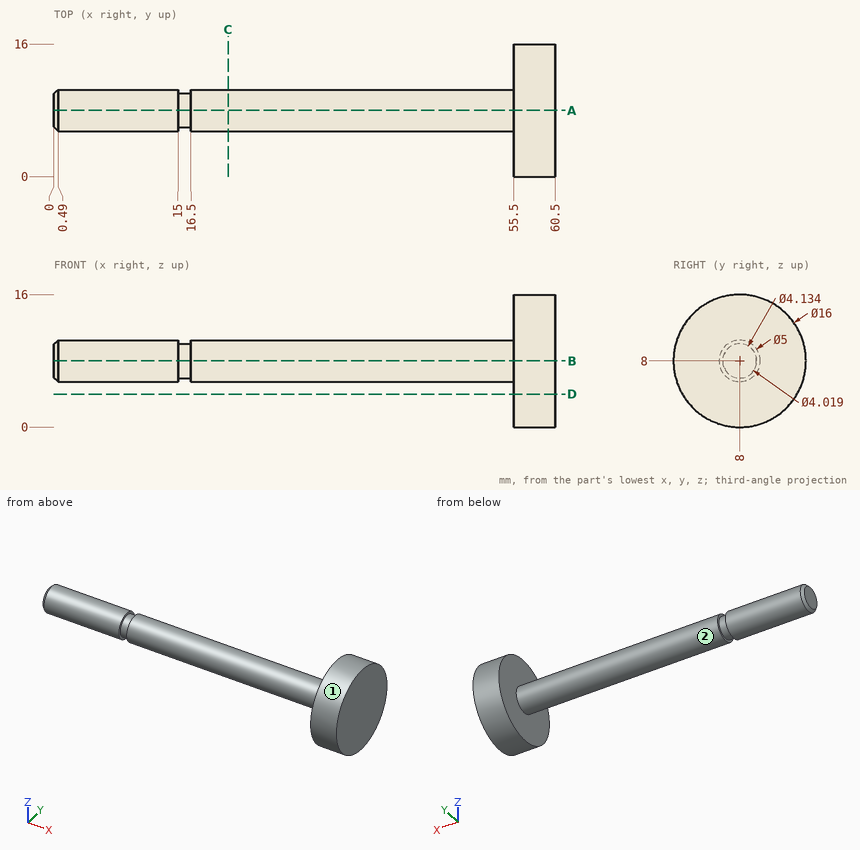
Check sheet for the drawn part. Datum: minimum x, y, z corner. Units: mm. A direction names the side the tool comes from. Give positions to 0.01 mm unless a question says otherwise; leave off trailing zeros. Write each loop counter-clockwise with the first axis right and the second up, starting at its lowest first coordinate (ties: lowest second). Pieces come first, ordered by that corner, then holes.
(1) Gauge pin test, flat ends, axial feed: pin 1 (6 mm diameter, centred on y = 3.5, z = 12, fed in from -X); pin 2 (3 mm diameter, centred on x = 38.5, y = 10.5, fed in from +Z); pin 3 (6 mm diameter, centred on x = 38, z = 10, fed in from +Y). Record the tip position at first contact, or that the pin passes through.
(2) Cross-section at C-C (x = 21). Enter the section's corners in (y, z).
(3) Cross-section at A-A (y = 8). Enter the section's corners in (x, z).
(4) Access from +Z, -Z, +X, -X, +Y, -Y to the whole of each face (thin tool, end or side, straight path). Record for the marked faces 1 and 2.
(5) Cross-section at D-D (z = 4). Enter the section's corners in (x, y).
(6) Material ranges on line 1 (X direction, y = 7.5, z = 0.75); line 2 (Y direction, x = 44, z = 9.5); line 3 (Y direction, x = 52.5, z = 7.25) (1 decimal), recorded low to high.
Worked out:
1. pin 1: stops at x = 55.5
1. pin 2: stops at z = 10.29
1. pin 3: stops at y = 10.5
2. outline: circle Ø5 at (8, 8)
3. outline: (0, 5.99) - (0.49, 5.5) - (15, 5.5) - (15, 5.93) - (16.5, 5.93) - (16.5, 5.5) - (55.5, 5.5) - (55.5, 0) - (60.5, 0) - (60.5, 16) - (55.5, 16) - (55.5, 10.5) - (16.5, 10.5) - (16.5, 10.07) - (15, 10.07) - (15, 10.5) - (0.49, 10.5) - (0, 10.01) - close
4. face 1: +X, -X
4. face 2: -X
5. outline: (55.5, 1.07) - (60.5, 1.07) - (60.5, 14.93) - (55.5, 14.93) - close
6. line 1: x = 55.5 to 60.5
6. line 2: y = 6 to 10
6. line 3: y = 5.6 to 10.4
